Verification items for this drawing (mm, ordinates from the low corner). Round coordinates to 2 decimals unless told otherwise and drop trailing zeros. Order: outer loops, then holes, each group sorted by start corner. A loop starts at its lowest first (then second) coordinate and runs counter-clockwise, first axis right, second up. Notation, with made-up numbers: (7, 57) -> (37, 57) arc R21 cw to (37, 68) -> close; hole circle Ø2 at (0, 61). An arc over 180 degrees is marked (long way). Put each result on its own line as item: value.
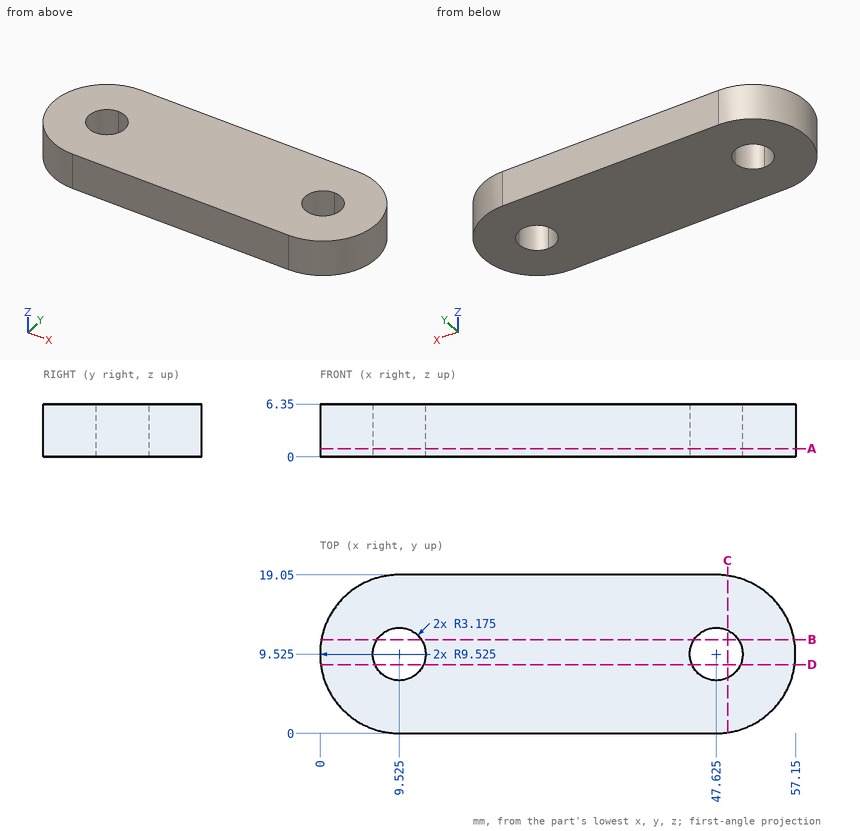
Item 1: Section check A-A on z = 1. Record the boundary of the cut face in (x, y) (3 decimals), then the cut area to 3 significant figures.
Check sheet entries:
outline: (9.525, 0) -> (47.625, 0) arc R9.525 ccw to (47.625, 19.05) -> (9.525, 19.05) arc R9.525 ccw to start; hole circle Ø6.35 at (9.525, 9.525); hole circle Ø6.35 at (47.625, 9.525)
area: 947 mm^2
Item 2: Section check C-C on x = 49. Record the boundary of the cut face in (y, z).
Check sheet entries:
outline: (0.1, 0) -> (6.66, 0) -> (6.66, 6.35) -> (0.1, 6.35) -> close; (12.39, 0) -> (18.95, 0) -> (18.95, 6.35) -> (12.39, 6.35) -> close
Item 3: Section check B-B on y = 11.25. Record the boundary of the cut face in (x, z).
Check sheet entries:
outline: (0.16, 0) -> (6.86, 0) -> (6.86, 6.35) -> (0.16, 6.35) -> close; (12.19, 0) -> (44.96, 0) -> (44.96, 6.35) -> (12.19, 6.35) -> close; (50.29, 0) -> (56.99, 0) -> (56.99, 6.35) -> (50.29, 6.35) -> close
Item 4: Material ranges on L1, parallel to X at y = 8.25, z = 1.25; L2, parallel to X at y = 7.5, z = 5.5; L3, parallel to Y at x = 9, z = 6, recorded low to high. Write a range as [from, to].
Check sheet entries:
L1: x = [0.09, 6.62], [12.43, 44.72], [50.53, 57.06]
L2: x = [0.22, 7.08], [11.97, 45.18], [50.07, 56.93]
L3: y = [0.01, 6.39], [12.66, 19.04]
Item 5: Gauge pin test, flat end, axial feed: pin 1 Ø2 at (y, z) = (12, 4.5) entering from -X. Record the tip position at first contact, or that the pin passes through.
Check sheet entries:
pin 1: stops at x = 0.11
Item 6: Section check D-D on y = 8.25. Record the boundary of the cut face in (x, z), then the cut area to 3 significant figures.
Check sheet entries:
outline: (0.09, 0) -> (6.62, 0) -> (6.62, 6.35) -> (0.09, 6.35) -> close; (12.43, 0) -> (44.72, 0) -> (44.72, 6.35) -> (12.43, 6.35) -> close; (50.53, 0) -> (57.06, 0) -> (57.06, 6.35) -> (50.53, 6.35) -> close
area: 288 mm^2
